```python
from build123d import *

# Parameters (mm, degrees)
SKETCH_1_W               = 5
SKETCH_1_H               = 4
EXTRUDE_1_DEPTH          = 0.2
LOFT_3_OUTLINE_W         = 4.8
LOFT_3_OUTLINE_H         = 3.8
LOFT_3_DEPTH             = 0.6
LOFT_3_DRAFT             = -9.4623222
SKETCH_9_W               = 0.5
SKETCH_9_H               = 0.2
PATTERN_LINEAR_1_COUNT   = 2
PATTERN_LINEAR_1_PITCH   = 2.54
MIRROR_1_COPY_1_SKETCH_W = 0.5
MIRROR_1_COPY_1_SKETCH_H = 0.2


# Read off the part's stored shape, not the designer's step: 放样3
with BuildPart() as part:
    # 草图1 → 凸台-拉伸1 (new body)
    with BuildSketch(Plane(origin=(0, 0, 0), x_dir=(1, 0, 0), z_dir=(0, 1, 0))):
        with Locations((2.5, 2)):
            Rectangle(SKETCH_1_W, SKETCH_1_H)
    extrude(amount=EXTRUDE_1_DEPTH)


with BuildPart() as loft_3_tool:
    # 放样3 outline → 放样3 (with draft: the straight prism first)
    with BuildSketch(Plane(origin=(0, -0.6, 0), x_dir=(1, 0, 0), z_dir=(0, 1, 0))):
        with Locations((2.5, 2)):
            Rectangle(LOFT_3_OUTLINE_W, LOFT_3_OUTLINE_H)
    extrude(amount=LOFT_3_DEPTH)
    # 放样3: the draft: its side faces are tilted about the plane it starts from
    loft_3_sides = [loft_3_tool.faces().sort_by_distance(p)[0] for p in [
        (2.5, -0.3, -3.9),
        (0.1, -0.3, -2),
        (2.5, -0.3, -0.1),
        (4.9, -0.3, -2),
    ]]
    draft(loft_3_sides, Plane(origin=(0, -0.6, 0), x_dir=(1, 0, 0), z_dir=(0, 1, 0)), LOFT_3_DRAFT)


with BuildPart() as part_1:
    add(part.part)

    # 放样3: add loft_3_tool
    add(loft_3_tool.part)

    # 草图4 → 放样5 section 0
    with BuildSketch(Plane(origin=(0, 0.2, 0), x_dir=(1, 0, 0), z_dir=(0, 1, 0))):
        with BuildLine():
            Line((0, 4), (5, 4))
            Line((5, 4), (5, 0))
            Line((5, 0), (0, 0))
            Line((0, 0), (0, 4))
        make_face()
    # 草图3 → 放样5 section 1
    with BuildSketch(Plane(origin=(0, 1.9, 0), x_dir=(1, 0, 0), z_dir=(0, 1, 0))):
        with BuildLine():
            Line((0.15, 3.85), (4.85, 3.85))
            Line((4.85, 3.85), (4.85, 0.15))
            Line((4.85, 0.15), (0.15, 0.15))
            Line((0.15, 0.15), (0.15, 3.85))
        make_face()
    loft()

    # 草图6 → 旋转1 (revolve)
    with BuildSketch(Plane(origin=(0, 1.9, 0), x_dir=(1, 0, 0), z_dir=(0, 1, 0))):
        with BuildLine():
            Line((1.65, 3.85), (1.65, 0.15))
            add(Edge.make_bspline(
                [(1.65, 3.85), (0.15, 3.85), (0.15, 2), (0.15, 0.15), (1.65, 0.15)],
                knots=[0, 0, 0, 1.570796327, 1.570796327, 3.141592654, 3.141592654, 3.141592654], degree=2, weights=[1, 0.707106781, 1, 0.707106781, 1]))
        make_face()
    revolve(axis=Axis((1.65, 1.9, 0.373474455), (0, 0, -1)))

    # 扫描2: sweep along a path in 草图7
    with BuildLine(Plane(origin=(3.77, 0, 0), x_dir=(0, 0, -1), z_dir=(1, 0, 0))) as sweep_2_path:
        Line((0, 0.099936428), (-0.484226547, 0.099936428))
        ThreePointArc((-0.484226547, 0.099936428), (-0.610923653, 0.059163591), (-0.690061218, -0.047849619))
        Line((-0.690061218, -0.047849619), (-0.770446454, -0.286097268))
        ThreePointArc((-0.770446454, -0.286097268), (-0.852673785, -0.402517912), (-0.98520599, -0.45496136))
        Line((-0.98520599, -0.45496136), (-1.5, -0.5))
    # 草图9 → 扫描2 (sweep)
    with BuildSketch(Plane.XY.offset(1.5)):
        with Locations((3.77, -0.5)):
            Rectangle(SKETCH_9_W, SKETCH_9_H)
    sweep_2 = sweep(path=sweep_2_path.line)

    # 阵列(线性)1: 扫描2 ×2
    with Locations(*[(-i * PATTERN_LINEAR_1_PITCH, 0, 0) for i in range(1, PATTERN_LINEAR_1_COUNT)]):
        add(sweep_2)

    # 镜向1: 扫描2 across plane
    add(sweep_2.mirror(Plane.XY.offset(-2)))

    # 镜向1 copy 1: sweep along a path in 镜向1 copy 1 path
    with BuildLine(Plane(origin=(1.23, 0, -4), x_dir=(0, 0, 1), z_dir=(1, 0, 0))) as mirror_1_copy_1_path:
        Line((0, -0.099936428), (-0.484226547, -0.099936428))
        ThreePointArc((-0.484226547, -0.099936428), (-0.610923653, -0.059163591), (-0.690061218, 0.047849619))
        Line((-0.690061218, 0.047849619), (-0.770446454, 0.286097268))
        ThreePointArc((-0.770446454, 0.286097268), (-0.852673785, 0.402517912), (-0.98520599, 0.45496136))
        Line((-0.98520599, 0.45496136), (-1.5, 0.5))
    # 镜向1 copy 1 sketch → 镜向1 copy 1 (sweep)
    with BuildSketch(Plane(origin=(-2.54, 0, -5.5), x_dir=(1, 0, 0), z_dir=(0, 0, -1))):
        with Locations((3.77, 0.5)):
            Rectangle(MIRROR_1_COPY_1_SKETCH_W, MIRROR_1_COPY_1_SKETCH_H)
    sweep(path=mirror_1_copy_1_path.line)


solid = part_1.part
```
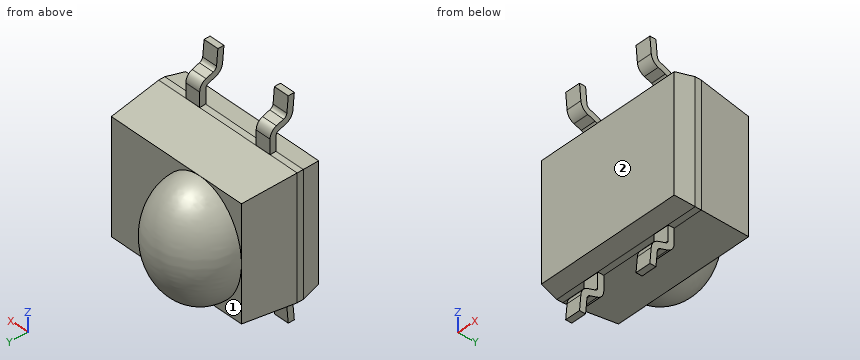
Design review of the part built by this model. Coordinates are the model's own, in mm. Face numbers are marked on the shaded views. A direction names the side the tool comes from. Coordinates: 2 decimals unless noted, no trailing zeros. One line per question, with ' | ' between items.
(1) For pin 1 Ø1 at (x, z) = (4, -2) entering from +Y; pin 2 Ø1 at (y, z) = (2.5, 0.5) entering from +X; pin 3 Ø2 at (x, y) = (2.5, 2) entering from -Z; pin 4 Ø1.7 at (x, z) = (1, -1) entering from +Y, all flat-tipped, find the tip position at first contact; note any pin that passes through.
Filled in:
pin 1: stops at y = 1.9 | pin 2: passes through | pin 3: stops at z = -3.93 | pin 4: stops at y = 3.37
(2) Machinability: for the marked faces 1 and 2, which of the approach directions +Z, -Z, +X, -X, +Y, -Y give a long, thin tool a straight path to every point of the face, cutting with its end or side? Answer none if there is none.
Filled in:
face 1: -Z, -X, +Y | face 2: +Z, -Z, +X, -X, -Y
(3) Wall thickness on probe 1 along Y at (x, z) = (0.5, -3.5); probe 2 along Y at (x, z) = (0.85, -2.25); probe 3 along Z at (x, y) = (2.15, 0.8): over which ranges is each line inside the solid? List them lowest first.
Filled in:
probe 1: y = -0.6 to 1.9 | probe 2: y = -0.6 to 3.15 | probe 3: z = -3.95 to -0.05
